Here's how the part is built. I have some questions about the finished solid (model axes, mm). A direction names the side the tool comes from. Round coordinates to 2 decimals unless told otherwise and drop trailing zeros. Order: outer loops, then holes, each group sorted by start corner. A loop starts at its lowest first (then second) coordinate and runs counter-clockwise, first axis right, second up. Notation, with made-up numbers: (49.5, 25) -> (93.5, 25) arc R16 cw to (93.5, 49) -> close; hole circle Ø3 at (-24.5, 72.25). An arc over 180 degrees is marked (long way). Answer in a Markdown table with one row per item.
```python
from build123d import *

# Parameters (mm, degrees)
EXTRUDE_THIN1_DEPTH = 25.4
FILLET1_R           = 3.175
SKETCH2_R           = 3.175
CUT_EXTRUDE1_DEPTH  = 58.589283942
SKETCH3_R           = 3.175
CUT_EXTRUDE2_DEPTH  = 60.56828015


with BuildPart() as part:
    # Sketch1 → Extrude-Thin1 (new, symmetric)
    with BuildSketch(Plane(origin=(0, 0, 0), x_dir=(1, 0, 0), z_dir=(0, 1, 0))):
        Polygon((0, 38.1), (0, 0), (38.1, 0), (38.1, 3.175), (3.175, 3.175), (3.175, 38.1), align=None)
    extrude(amount=EXTRUDE_THIN1_DEPTH, both=True)

    # Fillet1
    fillet1_edges = [part.edges().sort_by_distance(p)[0] for p in [
        (3.175, 0, -3.175),
        (38.1, 0, -3.175),
        (3.175, 0, -38.1),
    ]]
    fillet(fillet1_edges, radius=FILLET1_R - 0.0001)  # a hair under: the kernel refuses the full size

    # Sketch2 → Cut-Extrude1 (cut, through all)
    with BuildSketch(Plane(origin=(0, 0, -3.175), x_dir=(-1, 0, 0), z_dir=(0, 0, -1))):
        with Locations((-19.05, 12.7)):
            Circle(SKETCH2_R)
        with Locations((-19.05, -12.7)):
            Circle(SKETCH2_R)
    extrude(amount=-CUT_EXTRUDE1_DEPTH, mode=Mode.SUBTRACT)

    # Sketch3 → Cut-Extrude2 (cut, through all)
    with BuildSketch(Plane.ZY):
        with Locations((-19.05, 12.7)):
            Circle(SKETCH3_R)
        with Locations((-19.05, -12.7)):
            Circle(SKETCH3_R)
    extrude(amount=-CUT_EXTRUDE2_DEPTH, mode=Mode.SUBTRACT)


solid = part.part
```
1. For pin 1 Ø1 at (x, y) = (11, -20) entering from -Z (3 decimals); pin 2 Ø6 at (y, z) = (-3.5, -31.5) entering from +X (3 decimals); pin 3 Ø8.5 at (x, y) = (19.05, -12.7) entering from +Z; pin 4 Ø6 at (x, y) = (8.5, -20) entering from -Z, each with a flat end and sliding along its axis, tell me the tip position at first contact or that it passes through.
Numbers:
| item | result |
|---|---|
| pin 1 | stops at z = -3.175 |
| pin 2 | stops at x = 3.175 |
| pin 3 | stops at z = 0 |
| pin 4 | stops at z = -3.29 |
2. For faces 4 (the face through (0, 0, -19)), 5 (the face through (3.175, 0, -20)), which set-ups out of +Z, -Z, +X, -X, +Y, -Y let a thin tool reach every point of the face, with its end or its side?
Numbers:
| item | result |
|---|---|
| face 4 | +Z, -Z, -X, +Y, -Y |
| face 5 | -Z, +X, +Y, -Y |
3. We'd pull the mould along Z, two halves only. Please class faces 1 (the face through (1.565, -15.517, -17.585)), 2 (the face through (21, 0, -3.175)), 3 (the face through (17.585, -15.517, -1.61)): released by +Z, released by -Z, zero draft, split by the parting line, or undercut.
Numbers:
| item | result |
|---|---|
| face 1 | undercut |
| face 2 | released by -Z |
| face 3 | zero draft |
4. Suppose I cut it at B-B on x = 19.05. Write out the boundary of the cut face in (y, z) (3 decimals).
Numbers:
| item | result |
|---|---|
| outline | (-25.4, -3.175) -> (-15.875, -3.175) -> (-15.875, 0) -> (-25.4, 0) -> close; (-9.525, -3.175) -> (9.525, -3.175) -> (9.525, 0) -> (-9.525, 0) -> close; (15.875, -3.175) -> (25.4, -3.175) -> (25.4, 0) -> (15.875, 0) -> close |
5. Please list where these lines run through material, in increasing order: line 1 along Y through (x, z) = (1, -19); line 2 along Z through (x, y) = (29.5, -3) (3 decimals); line 3 along X through (y, z) = (6.5, -13) (3 decimals).
Numbers:
| item | result |
|---|---|
| line 1 | y = -25.4 to -15.87, -9.53 to 9.53, 15.87 to 25.4 |
| line 2 | z = -3.175 to 0 |
| line 3 | x = 0 to 3.175 |
6. Suppose I cut it at C-C on z = -19.05. Write out the boundary of the cut face in (x, y) (3 decimals).
Numbers:
| item | result |
|---|---|
| outline | (0, -25.4) -> (3.175, -25.4) -> (3.175, -15.875) -> (0, -15.875) -> close; (0, -9.525) -> (3.175, -9.525) -> (3.175, 9.525) -> (0, 9.525) -> close; (0, 15.875) -> (3.175, 15.875) -> (3.175, 25.4) -> (0, 25.4) -> close |
7. Suppose I cut it at A-A on y = 12.7. State how many separate pieces and enclosed holes the cut face has, then the cut area to 3 significant figures.
Numbers:
| item | result |
|---|---|
| separate pieces | 3 |
| enclosed holes | 0 |
| area | 189 mm2 |
